from build123d import *

# Parameters (mm, degrees)
BOSS_EXTRUDE1_DEPTH = 9
CHAMFER1_SIZE       = 1
SKETCH2_R           = 2
CUT_EXTRUDE1_DEPTH  = 7
SKETCH3_R           = 3
CUT_EXTRUDE2_DEPTH  = 20.5


with BuildPart() as part:
    # Sketch1 → Boss-Extrude1 (new body)
    with BuildSketch(Plane.XY):
        with BuildLine():
            Line((-0.75, 21), (0.75, 21))
            Line((0.75, 21), (0.75, 17.483921185))
            ThreePointArc((0.75, 17.483921185), (17.5, 0), (0.75, -17.483921185))
            Line((0.75, -17.483921185), (0.75, -26.489384666))
            ThreePointArc((0.75, -26.489384666), (0, 26.5), (-0.75, -26.489384666))
            Line((-0.75, -26.489384666), (-0.75, -17.483921185))
            ThreePointArc((-0.75, -17.483921185), (-17.5, 0), (-0.75, 17.483921185))
            Line((-0.75, 17.483921185), (-0.75, 21))
        make_face()
    extrude(amount=BOSS_EXTRUDE1_DEPTH)

    # Chamfer1
    chamfer1_edges = [part.edges().sort_by_distance(p)[0] for p in [
        (0, 26.5, 0),
        (17.5, 0, 0),
        (0, 26.5, 9),
        (-17.5, 0, 9),
        (17.5, 0, 9),
        (-17.5, 0, 0),
    ]]
    chamfer(chamfer1_edges, length=CHAMFER1_SIZE)

    # Sketch2 → Cut-Extrude1 (cut, symmetric)
    with BuildSketch(Plane(origin=(0, 0, 0), x_dir=(0, 0, -1), z_dir=(1, 0, 0))):
        with Locations((-4.5, -22)):
            Circle(SKETCH2_R)
    extrude(amount=CUT_EXTRUDE1_DEPTH, both=True, mode=Mode.SUBTRACT)

    # Sketch3 → Cut-Extrude2 (cut, through all)
    with BuildSketch(Plane(origin=(7, 0, 0), x_dir=(0, 0, -1), z_dir=(1, 0, 0))):
        with Locations((-4.5, -22)):
            Circle(SKETCH3_R)
    cut_extrude2 = extrude(amount=CUT_EXTRUDE2_DEPTH, mode=Mode.SUBTRACT)

    # Mirror1: Cut-Extrude2 across plane
    add(cut_extrude2.mirror(Plane(origin=(0, 0, 0), x_dir=(0, 0, 1), z_dir=(1, 0, 0))), mode=Mode.SUBTRACT)


solid = part.part
The model under review builds one solid part; all positions refer to its coordinate system, in mm. A direction names the side the tool comes from. Give positions to 0.01 mm unless a question says otherwise; leave off trailing zeros. Loops run counter-clockwise (first coordinate to the right, second up) from the corner with the lowest first, then second, coordinate; pieces in that order, holes last. Notation, with made-up numbers: (64, 70.25) -> (110, 70.25) arc R16 ccw to (110, 76.25) -> close; hole circle Ø1 at (57.25, 23). An arc over 180 degrees is marked (long way). Put each result on its own line as item: value. Start each with the question number.
1. For faces 5 (the face through (-11.381, -19.026, 4.891)), 6 (the face through (0.75, -22, 2)), 7 (the face through (11.381, -19.026, 4.891)), list the 3-axis set-ups (+Z, -Z, +X, -X, +Y, -Y) from which the entire face can be reached by the end or side of a thin tool; tool diameter is ignored.
2. We need section B-B on z = 3.5. State the section outline as (x, y) points.
3. We need section A-A on y = 0. State the section outline as (x, z) points, then the cut area to 3 significant figures.
4. Clearance check with flat-ended pins moving along their axes: P1, Ø3.5, axis at y = -22, z = 4.5, coming from the +X side; P2, Ø4, axis at x = -7.5, z = 4.5, coming from the -Y side; P3, Ø3, axis at y = 20, z = 2.5, coming from the +X side; P4, Ø1.1, axis at y = 19.5, z = 4, coming from the -X side. State where each tip first meets the part, or that it passes through.
5. Mouldability with a two-part tool opening along Y and no side actions: class faces 1 (the face through (0.75, 19, 4)), 2 (the face through (-3.831, -20.017, 4.76)), 3 (the face through (-7, -22, 7)), 4 (the face through (0, 21, 4)) as released by +Y, released by -Y, zero draft, split by the parting line, or undercut.
6. Wall thickness on probe 1 along Z at (x, y) = (-9, -22); probe 2 along Y at (x, z) = (4, 4.5); probe 3 along X at (y, z) = (-21, 6.75): over which ranges is each line inside the solid? List them lowest first.
7. We need section C-C on x = -6. State how many separate pieces and enclosed holes the cut face has, then the cut area to 3 significant figures.
Determined:
1. face 5: -X
1. face 6: +Z, -Z, -Y
1. face 7: +X
2. outline: (-18.29, -19.17) -> (-7, -19.17) -> (-7, -20.27) -> (-0.75, -20.27) -> (-0.75, -17.48) arc R17.5 cw to (-0.75, 17.48) -> (-0.75, 21) -> (0.75, 21) -> (0.75, 17.48) arc R17.5 cw to (0.75, -17.48) -> (0.75, -20.27) -> (7, -20.27) -> (7, -19.17) -> (18.29, -19.17) arc R26.5 ccw (long way) to start; (-9.26, -24.83) arc R26.5 ccw to (-0.75, -26.49) -> (-0.75, -23.73) -> (-7, -23.73) -> (-7, -24.83) -> close; (0.75, -26.49) arc R26.5 ccw to (9.26, -24.83) -> (7, -24.83) -> (7, -23.73) -> (0.75, -23.73) -> close
3. outline: (-26.5, 1) -> (-25.5, 0) -> (-18.5, 0) -> (-17.5, 1) -> (-17.5, 8) -> (-18.5, 9) -> (-25.5, 9) -> (-26.5, 8) -> close; (17.5, 1) -> (18.5, 0) -> (25.5, 0) -> (26.5, 1) -> (26.5, 8) -> (25.5, 9) -> (18.5, 9) -> (17.5, 8) -> close
3. area: 158 mm^2
4. P1: through
4. P2: y = -25.92
4. P3: x = 18.97
4. P4: x = -18.52
5. face 1: zero draft
5. face 2: undercut
5. face 3: undercut
5. face 4: released by -Y
6. probe 1: 0 to 1.5, 7.5 to 9
6. probe 2: -26.2 to -24, -20 to -17.04, 17.04 to 26.2
6. probe 3: -7 to -0.75, 0.75 to 7
7. separate pieces: 2
7. enclosed holes: 1
7. area: 152 mm^2
